CAD build for the part. Positions are in the model's coordinates, mm. A direction names the side the tool comes from. Round coordinates to 2 decimals unless told otherwise and drop trailing zeros. Loops run counter-clockwise (first coordinate to the right, second up) from the corner with the lowest first, then second, coordinate; pieces in that order, holes last.
```python
from build123d import *

# Parameters (mm, degrees)
SKETCH1_R                   = 60.6425
SKETCH1_R_2                 = 57.4675
BOSS_EXTRUDE1_DEPTH         = 50.8
BOSS_EXTRUDE2_START         = -26.9875
SKETCH2_R                   = 76.2
SKETCH2_R_2                 = 60.6425
BOSS_EXTRUDE2_DEPTH         = 3.175
F_1_4_CLEARANCE_HOLE1_D     = 6.5278
F_1_4_CLEARANCE_HOLE1_DEPTH = 38.354
F_1_4_CLEARANCE_HOLE1_TIP   = 1.961148974


with BuildPart() as part:
    # Sketch1 → Boss-Extrude1 (new body)
    with BuildSketch(Plane(origin=(0, 0, 0), x_dir=(1, 0, 0), z_dir=(0, 1, 0))):
        with Locations(Location((0, 0, 0), (0, 0, 270))):
            Circle(SKETCH1_R)
        with Locations(Location((0, 0, 0), (0, 0, 270))):
            Circle(SKETCH1_R_2, mode=Mode.SUBTRACT)
    extrude(amount=BOSS_EXTRUDE1_DEPTH)

    # Sketch2 → Boss-Extrude2 (add)
    with BuildSketch(Plane(origin=(0, 50.8, 0), x_dir=(1, 0, 0), z_dir=(0, 1, 0)).offset(BOSS_EXTRUDE2_START)):
        with Locations(Location((0, 0, 0), (0, 0, 270))):
            Circle(SKETCH2_R)
        with Locations(Location((0, 0, 0), (0, 0, 270))):
            Circle(SKETCH2_R_2, mode=Mode.SUBTRACT)
    extrude(amount=BOSS_EXTRUDE2_DEPTH)

    # 1/4 Clearance Hole1
    with Locations(Plane(origin=(0, 26.9875, 0), x_dir=(1, 0, 0), z_dir=(0, 1, 0))):
        with Locations((-68.42125, 0)):
            Hole(F_1_4_CLEARANCE_HOLE1_D / 2, depth=F_1_4_CLEARANCE_HOLE1_DEPTH)
            with Locations((0, 0, -(F_1_4_CLEARANCE_HOLE1_DEPTH + F_1_4_CLEARANCE_HOLE1_TIP / 2))):  # 118° drill point
                Cone(0, F_1_4_CLEARANCE_HOLE1_D / 2, F_1_4_CLEARANCE_HOLE1_TIP, mode=Mode.SUBTRACT)


solid = part.part
```
Item 1: 3-axis set-ups, long thin cutter, end or side, ignore diameter. For faces 1 (the flat face through (-22, 26.987, -57)), 2 (the cylindrical face through (-46.367, 25.378, -60.47)), 3 (the cylindrical face through (-53.8, 11.74, 27.98)): which of +Z, -Z, +X, -X, +Y, -Y reach the whole face in a straight line?
Answers follow:
face 1: +Y
face 2: +Y, -Y
face 3: -Y
Item 2: Cut at C-C, the plane z = -16. Give the cut face in (x, y), plus the area to 3 significant figures.
Answers follow:
outline: (-74.5, 23.81) - (-58.49, 23.81) - (-58.49, 0) - (-55.2, 0) - (-55.2, 50.8) - (-58.49, 50.8) - (-58.49, 26.99) - (-74.5, 26.99) - close; (55.2, 0) - (58.49, 0) - (58.49, 23.81) - (74.5, 23.81) - (74.5, 26.99) - (58.49, 26.99) - (58.49, 50.8) - (55.2, 50.8) - close
area: 437 mm2
Item 3: Cut at A-A, the plane z = 0. Give the cut face in (x, y).
Answers follow:
outline: (-76.2, 23.81) - (-71.69, 23.81) - (-71.69, 26.99) - (-76.2, 26.99) - close; (-65.16, 23.81) - (-60.64, 23.81) - (-60.64, 0) - (-57.47, 0) - (-57.47, 50.8) - (-60.64, 50.8) - (-60.64, 26.99) - (-65.16, 26.99) - close; (57.47, 0) - (60.64, 0) - (60.64, 23.81) - (76.2, 23.81) - (76.2, 26.99) - (60.64, 26.99) - (60.64, 50.8) - (57.47, 50.8) - close
Item 4: Flat gauge pins, fed straight in: P1, Ø1.5, axis at x = 7, y = 14, coming from the -Z side; P2, Ø5, axis at y = 43, z = 10.5, coming from the +X side; P3, Ø12, axis at y = 45.5, z = 46.5, coming from the +X side. Where does each tip first touch, or does it go through?
Answers follow:
P1: stops at z = -60.32
P2: stops at x = 60.11
P3: stops at x = 45.14
Item 5: Probe line 1 (X direction, y = 31.5, z = -0.5); line 2 (Y direction, x = 60, z = -31.5); line 3 (X direction, y = 43, z = -26.5). List the from-to ranges inside material, lowest first.
Answers follow:
line 1: x = -60.64 to -57.47, 57.47 to 60.64
line 2: y = 23.81 to 26.99
line 3: x = -54.55 to -50.99, 50.99 to 54.55
Item 6: Cut at B-B, the plane x = 0. Give the cut face in (y, z).
Answers follow:
outline: (0, -60.64) - (23.81, -60.64) - (23.81, -76.2) - (26.99, -76.2) - (26.99, -60.64) - (50.8, -60.64) - (50.8, -57.47) - (0, -57.47) - close; (0, 57.47) - (50.8, 57.47) - (50.8, 60.64) - (26.99, 60.64) - (26.99, 76.2) - (23.81, 76.2) - (23.81, 60.64) - (0, 60.64) - close
Item 7: Cut at D-D, the plane x = -67. Give the cut face in (y, z).
Answers follow:
outline: (23.81, -36.3) - (26.99, -36.3) - (26.99, -2.94) - (23.81, -2.94) - close; (23.81, 2.94) - (26.99, 2.94) - (26.99, 36.3) - (23.81, 36.3) - close
Item 8: Two-plate mould, pull along X, no slides. Class faces 4 (the flat face through (-22, 23.812, -57)), 5 (the cylindrical face through (-53.8, 38.73, 27.98)), 6 (the cylindrical face through (-65.16, 25.38, -0.14)): released by +X, released by -X, zero draft, split by the parting line, or undercut.
Answers follow:
face 4: zero draft
face 5: split by the parting line
face 6: undercut
